Part model, mm, in its own coordinate system. A direction names the side the tool comes from. Give positions to 0.01 mm unless a question says otherwise; leave off trailing zeros. Loops run counter-clockwise (first coordinate to the right, second up) from the corner with the lowest first, then second, coordinate; pieces in that order, holes last. Notation, with made-up numbers: (43.5, 62) -> (87.5, 62) arc R22 ccw to (87.5, 91) -> close; hole circle Ø5 at (32.25, -32). An arc over 180 degrees is marked (long way). One line per question, with ' | ' between items.
```python
from build123d import *

# Parameters (mm, degrees)
SKETCH1_R           = 6
BOSS_EXTRUDE2_DEPTH = 20
SKETCH3_R           = 10
BOSS_EXTRUDE3_DEPTH = 3
FILLET1_R           = 10
FILLET2_R           = 10


with BuildPart() as part:
    # Sketch1 → Boss-Extrude2 (new body)
    with BuildSketch(Plane.XY):
        with BuildLine():
            Line((-70, 20), (70, 20))
            ThreePointArc((70, 20), (90, 0), (70, -20))
            Line((70, -20), (-70, -20))
            ThreePointArc((-70, -20), (-90, 0), (-70, 20))
        make_face()
        with Locations((-70, 0)):
            Circle(SKETCH1_R, mode=Mode.SUBTRACT)
        with Locations((70, 0)):
            Circle(SKETCH1_R, mode=Mode.SUBTRACT)
    extrude(amount=BOSS_EXTRUDE2_DEPTH)

    # Sketch3 → Boss-Extrude3 (add)
    with BuildSketch(Plane.XY):
        with Locations((-70, 0)):
            Circle(SKETCH3_R)
        with Locations((70, 0)):
            Circle(SKETCH3_R)
    extrude(amount=BOSS_EXTRUDE3_DEPTH)

    # Fillet1
    fillet1_edges = [part.edges().sort_by_distance(p)[0] for p in [
        (90, 0, 20),
        (0, 20, 20),
        (-90, 0, 20),
        (0, -20, 20),
    ]]
    fillet(fillet1_edges, radius=FILLET1_R)

    # Fillet2
    fillet2_edges = [part.edges().sort_by_distance(p)[0] for p in [
        (90, 0, 0),
        (0, -20, 0),
        (-90, 0, 0),
        (0, 20, 0),
    ]]
    fillet(fillet2_edges, radius=FILLET2_R - 0.0001)  # a hair under: the kernel refuses the full size


solid = part.part
```
1) Saw through at B-B (z = 7.75). Give the cut face in (x, y).
Found:
outline: (-70, -19.74) -> (70, -19.74) arc R19.74 ccw to (70, 19.74) -> (-70, 19.74) arc R19.74 ccw to start; hole circle Ø12 at (-70, 0); hole circle Ø12 at (70, 0)
2) Drill centre lines: line 1 (X direction, y = 0, z = 16); line 2 (X direction, y = 4, z = 5.75); line 3 (Y direction, x = 70, z = 16.5). Where is each one in solid material? Low to high.
Found:
line 1: -88 to -76, -64 to 64, 76 to 88 | line 2: -88.63 to -74.47, -65.53 to 65.53, 74.47 to 88.63 | line 3: -17.6 to -6, 6 to 17.6
3) Pull direction X, two halves, no side cores. Call faces 1 (the cylindrical face through (0.98, 17.15, 16.99)), 2 (the flat face through (70, 0, 3)): pulls with the +X half, pulls with the -X half, needs draft (parallel to the pull), parting line crosses it, or undercut.
Found:
face 1: needs draft | face 2: undercut
4) Tool access for faces 3 (the flat face through (1, 0, 0)), 4 (the flat face through (-70, 0, 3)): list every direction of +Z, -Z, +X, -X, +Y, -Y with a clear straight run to the whole face (end or side of a thin tool).
Found:
face 3: -Z, +X, -X, +Y, -Y | face 4: +Z
5) Pin check, flat tips, straight feed: P1, Ø1, axis at y = 12, z = 14, coming from the +X side; P2, Ø10, axis at y = -2.5, z = 16.5, coming from the +X side; P3, Ø1, axis at x = 32, y = -16, coming from the +Z side. Stop position of each tip, or through.
Found:
P1: x = 85.41 | P2: x = 89.82 | P3: z = 18.35
